Check sheet for the modelled part. Datum: model origin and axes. Units: mm. Coordinates: 2 decimals unless noted, no trailing zeros. Write each loop counter-clockwise with the first axis right and the second up, starting at its lowest first coordinate (ties: lowest second). Pieces come first, ordered by that corner, then holes. Notation, with made-up numbers: M -36,80 L 1,80 A21 ccw 1,117 Z; hole C 81.25,69 d4. An arc over 180 degrees is marked long. Answer as CSV lines item,"result". Start each with the question number.
1) Section check D-D (x = 20). Record the cut outline in (y, z).
2) Section check C-C (z = 10.5). Record the cut outline in (x, y), and give its area (3 significant figures).
3) Section check B-B (y = 0). Record the cut outline in (x, z).
4) Section check A-A (x = -20). Record the cut outline in (y, z), and give its area (3 significant figures).
5) Draft check along Y on faces 1 (the cylindrical face through (-40.72, 30.49, 9.86)), 2 (the cylindrical face through (-40.49, -30.72, 9.86)), 3 (the flat face through (45, 0, 10)), 4 (the cylindrical face through (37.55, -7.28, 10.14)). Enter one of: +Y half, -Y half, draft (parallel to the pull), parting line (faces both ways), or undercut.
6) Material ranges on L1, parallel to X at y = -5, z = 9.5; L2, parallel to Y at x = -20, z = 5.5; L3, parallel to X at y = -12, z = 5, recorded low to high. Write a range as [from, to].
from build123d import *

# Parameters (mm, degrees)
BOSS_EXTRUDE1_DEPTH     = 20
SKETCH3_R               = 20
CUT_EXTRUDE2_DEPTH      = 1
CUT_EXTRUDE2_DEPTH_BACK = 21
SKETCH4_R               = 19
CUT_EXTRUDE3_DEPTH      = 21


with BuildPart() as part:
    # Sketch1 → Boss-Extrude1 (new body)
    with BuildSketch(Plane.XY):
        with BuildLine():
            Line((30, -35), (-30, -35))
            ThreePointArc((-30, -35), (-40.606601718, -30.606601718), (-45, -20))
            Line((-45, -20), (-45, 20))
            ThreePointArc((-45, 20), (-40.606601718, 30.606601718), (-30, 35))
            Line((-30, 35), (30, 35))
            ThreePointArc((30, 35), (40.606601718, 30.606601718), (45, 20))
            Line((45, 20), (45, -20))
            ThreePointArc((45, -20), (40.606601718, -30.606601718), (30, -35))
        make_face()
    extrude(amount=BOSS_EXTRUDE1_DEPTH)

    # Sketch3 → Cut-Extrude2 (cut, two sides)
    with BuildSketch(Plane.XY.offset(20)) as cut_extrude2_sk:
        with Locations((-20, 0)):
            Circle(SKETCH3_R)
    extrude(amount=CUT_EXTRUDE2_DEPTH, mode=Mode.SUBTRACT)
    extrude(cut_extrude2_sk.sketch, amount=-CUT_EXTRUDE2_DEPTH_BACK, mode=Mode.SUBTRACT)

    # Sketch4 → Cut-Extrude3 (cut, through all)
    with BuildSketch(Plane.XY.offset(20)):
        with Locations((20, 0)):
            Circle(SKETCH4_R)
    extrude(amount=-CUT_EXTRUDE3_DEPTH, mode=Mode.SUBTRACT)


solid = part.part
Results found:
1,outline,"M -35,0 L -19,0 L -19,20 L -35,20 Z; M 19,0 L 35,0 L 35,20 L 19,20 Z"
2,outline,"M -45,-20 A15 ccw -30,-35 L 30,-35 A15 ccw 45,-20 L 45,20 A15 ccw 30,35 L -30,35 A15 ccw -45,20 Z; hole C -20,0 d40; hole C 20,0 d38"
2,area,"3,720 mm2"
3,outline,"M -45,0 L -40,0 L -40,20 L -45,20 Z; M 0,0 L 1,0 L 1,20 L 0,20 Z; M 39,0 L 45,0 L 45,20 L 39,20 Z"
4,outline,"M -35,0 L -20,0 L -20,20 L -35,20 Z; M 20,0 L 35,0 L 35,20 L 20,20 Z"
4,area,"600 mm2"
5,face 1,"+Y half"
5,face 2,"-Y half"
5,face 3,"draft"
5,face 4,"undercut"
6,L1,"x = [-45, -39.36], [-0.64, 1.67], [38.33, 45]"
6,L2,"y = [-35, -20], [20, 35]"
6,L3,"x = [-45, -36], [-4, 5.27], [34.73, 45]"
